```python
from build123d import *

# Parameters (mm, degrees)
SKETCH1_W           = 25.4
SKETCH1_H           = 95.25
SKETCH1_R           = 3.175
SKETCH1_W_2         = 11.1125
SKETCH1_H_2         = 31.75
BOSS_EXTRUDE1_DEPTH = 6.35
CUT_EXTRUDE1_DEPTH  = 99.782817332
FILLET1_R           = 1.27
FILLET2_R           = 5.55625


with BuildPart() as part:
    # Sketch1 → Boss-Extrude1 (new body)
    with BuildSketch(Plane(origin=(0, 0, 0), x_dir=(1, 0, 0), z_dir=(0, 1, 0))):
        with Locations((12.7, 47.625)):
            Rectangle(SKETCH1_W, SKETCH1_H)
        with Locations(Location((12.7, 82.55, 0), (0, 0, 270))):
            Circle(SKETCH1_R, mode=Mode.SUBTRACT)
        with Locations(Location((12.7, 12.7, 0), (0, 0, 270))):
            Circle(SKETCH1_R, mode=Mode.SUBTRACT)
        with Locations((12.7, 53.975)):
            Rectangle(SKETCH1_W_2, SKETCH1_H_2, mode=Mode.SUBTRACT)
    extrude(amount=BOSS_EXTRUDE1_DEPTH)

    # Sketch2 → Cut-Extrude1 (cut, through all)
    with BuildSketch(Plane(origin=(0, 6.35, 0), x_dir=(1, 0, 0), z_dir=(0, 1, 0))):
        with BuildLine():
            ThreePointArc((0, 82.549999981), (3.719743872, 91.530256114), (12.7, 95.25))
            Line((12.7, 95.25), (0, 95.25))
            Line((0, 95.25), (0, 82.549999981))
        make_face()
        with BuildLine():
            ThreePointArc((12.7, 95.25), (21.680256121, 91.530256121), (25.4, 82.55))
            Line((25.4, 82.55), (25.4, 95.25))
            Line((25.4, 95.25), (12.7, 95.25))
        make_face()
        with BuildLine():
            ThreePointArc((12.7, 0), (3.719743903, 3.719743855), (0, 12.699999932))
            Line((0, 12.699999932), (0, 0))
            Line((0, 0), (12.7, 0))
        make_face()
        with BuildLine():
            Line((25.4, 0), (25.4, 12.7))
            ThreePointArc((25.4, 12.7), (21.680256121, 3.719743879), (12.7, 0))
            Line((12.7, 0), (25.4, 0))
        make_face()
    extrude(amount=-CUT_EXTRUDE1_DEPTH, mode=Mode.SUBTRACT)

    # Fillet1
    fillet1_edges = [part.edges().sort_by_distance(p)[0] for p in [
        (25.4, 0, -47.625),
        (25.4, 6.35, -47.625),
        (0, 0, -47.624999957),
        (0, 6.35, -47.624999957),
        (12.69999999, 6.35, -95.25),
        (12.69999999, 0, -95.25),
        (12.700000034, 6.35, 0),
        (12.700000034, 0, 0),
    ]]
    fillet(fillet1_edges, radius=FILLET1_R)

    # Fillet2
    fillet2_edges = [part.edges().sort_by_distance(p)[0] for p in [
        (7.14375, 3.175, -38.1),
        (18.25625, 3.175, -38.1),
        (18.25625, 3.175, -69.85),
        (7.14375, 3.175, -69.85),
    ]]
    fillet(fillet2_edges, radius=FILLET2_R - 0.0001)  # a hair under: the kernel refuses the full size


solid = part.part
```
Geometry check sheet. Reference: the model listing, model coordinates, mm. A direction names the side the tool comes from. Round coordinates to 2 decimals unless told otherwise and drop trailing zeros. Loops run counter-clockwise (first coordinate to the right, second up) from the corner with the lowest first, then second, coordinate; pieces in that order, holes last. Notation, with made-up numbers: (-4, 78.5) - (26, 78.5) arc R20 ccw to (26, 100.5) - close; hole circle Ø2 at (87.25, 80). An arc over 180 degrees is marked (long way). Use a Markdown table: item, result.
Q1. Draft check along X on faces 1 (the flat face through (25.4, 3, -47)), 2 (the flat face through (18.256, 3, -54)), 3 (the flat face through (5, 6.35, -48)), 4 (the flat face through (0, 3, -47)). Enter one of: released by +X, released by -X, zero draft, split by the parting line, or undercut.
Solutions:
| item | result |
|---|---|
| face 1 | released by +X |
| face 2 | undercut |
| face 3 | zero draft |
| face 4 | released by -X |
Q2. Go/stop test with flat-tipped pins: P1, Ø5, axis at x = 9.5, z = -63, coming from the -Y side; P2, Ø1.5, axis at x = 21.5, y = 1, coming from the -Z side. Record where each tip stops, or that it passes through.
Solutions:
| item | result |
|---|---|
| P1 | stops at y = 0 |
| P2 | stops at z = -92.35 |
Q3. Cross-section at A-A on y = 2.5. State how many separate pieces and enclosed holes the cut face has, plus the area to 3 significant figures.
Solutions:
| item | result |
|---|---|
| separate pieces | 1 |
| enclosed holes | 3 |
| area | 1,890 mm2 |
Q4. Access from +Z, -Z, +X, -X, +Y, -Y to the whole of each face (thin tool, end or side, straight path). Record for faces 5 (the cylindrical face through (8.8, 3.2, -39.7)), 6 (the flat face through (5, 0, -48)).
Solutions:
| item | result |
|---|---|
| face 5 | +Y, -Y |
| face 6 | +Z, -Z, +X, -X, -Y |
Q5. Cross-section at D-D on z = -39.5. Record the cut outline in (x, y).
Solutions:
| item | result |
|---|---|
| outline | (0, 1.27) arc R1.27 ccw to (1.27, 0) - (9.01, 0) - (9.01, 6.35) - (1.27, 6.35) arc R1.27 ccw to (0, 5.08) - close; (16.39, 0) - (24.13, 0) arc R1.27 ccw to (25.4, 1.27) - (25.4, 5.08) arc R1.27 ccw to (24.13, 6.35) - (16.39, 6.35) - close |
Q6. Cross-section at B-B on z = -68. Record the cut outline in (x, y).
Solutions:
| item | result |
|---|---|
| outline | (0, 1.27) arc R1.27 ccw to (1.27, 0) - (8.56, 0) - (8.56, 6.35) - (1.27, 6.35) arc R1.27 ccw to (0, 5.08) - close; (16.84, 0) - (24.13, 0) arc R1.27 ccw to (25.4, 1.27) - (25.4, 5.08) arc R1.27 ccw to (24.13, 6.35) - (16.84, 6.35) - close |
Q7. Material ranges on line 1 (Z direction, x = 10.5, y = 5); line 2 (Z direction, x = 11, y = 2.5); line 3 (X direction, y = 3.75, z = -63), recorded low to high.
Solutions:
| item | result |
|---|---|
| line 1 | z = -95.06 to -84.84, -80.26 to -69.4, -38.55 to -14.99, -10.41 to -0.19 |
| line 2 | z = -95.14 to -85.23, -79.87 to -69.58, -38.37 to -15.38, -10.02 to -0.11 |
| line 3 | x = 0 to 7.14, 18.26 to 25.4 |
